Check sheet for the modelled part. Datum: model origin and axes. Units: mm. A direction names the side the tool comes from. Give positions to 0.01 mm unless a question says otherwise; leave off trailing zeros. Write each loop counter-clockwise with the first axis right and the second up, starting at its lowest first coordinate (ties: lowest second). Pieces come first, ordered by that corner, then holes.
from build123d import *

# Parameters (mm, degrees)
BOSS_EXTRUDE1_DEPTH = 12.625


with BuildPart() as part:
    # Sketch1 → Boss-Extrude1 (new, symmetric)
    with BuildSketch(Plane.XY):
        with BuildLine():
            Line((-600, 0), (0, 0))
            ThreePointArc((0, 0), (31, 31), (0, 62))
            Line((0, 62), (-20, 62))
            Line((-20, 62), (-20, 49.4))
            Line((-20, 49.4), (0, 49.4))
            ThreePointArc((0, 49.4), (18.4, 31), (0, 12.6))
            Line((0, 12.6), (-600, 12.6))
            Line((-600, 12.6), (-600, 0))
        make_face()
    extrude(amount=BOSS_EXTRUDE1_DEPTH, both=True)


solid = part.part
1) Sectioned sample at B-B on z = 7.5. Record the boundary of the cut face in (x, y), then the cut area to 3 significant figures.
2) Gauge pin test, flat ends, axial feed: pin 1 (14 mm diameter, centred on y = 58, z = 4.5, fed in from -X); pin 2 (12 mm diameter, centred on y = 35.5, z = 9.5, fed in from +X); pin 3 (1 mm diameter, centred on x = -153, z = -9, fed in from +Y); pin 4 (6 mm diameter, centred on x = -10, z = 1, fed in from -Y). Record the tip position at first contact, or that the pin passes through.
3) Scan lines: L1, parallel to Y at x = -1, z = 1.75; L2, parallel to X at y = 33, z = 7.5; L3, parallel to Y at x = -204.5, z = 4. Record each from-to range of solid material in increasing order.
4) Draft check along Y on faces 3 (the flat face through (-304, 0, 0)), 4 (the flat face through (-10, 49.4, 0)), 5 (the flat face through (-10, 62, 0)). Enter one of: +Y half, -Y half, draft (parallel to the pull), parting line (faces both ways), or undercut.
5) Access from +Z, -Z, +X, -X, +Y, -Y to the whole of each face (thin tool, end or side, straight path). Record for faces 1 (the cylindrical face through (30.993, 30.318, 0.177)), 2 (the flat face through (-20, 56, 0)).
6) Sectioned sample at A-A on x = -6.5. Record the boundary of the cut face in (y, z) (3 decimals).
7) Sectioned sample at C-C on y = 31. Record the boundary of the cut face in (x, z) (3 decimals), then the cut area to 3 significant figures.
8) Sectioned sample at D-D on x = -225. Record the boundary of the cut face in (y, z) (3 decimals).
Answers below:
1. outline: (-600, 0) - (0, 0) arc R31 ccw to (0, 62) - (-20, 62) - (-20, 49.4) - (0, 49.4) arc R18.4 cw to (0, 12.6) - (-600, 12.6) - close
1. area: 8,790 mm2
2. pin 1: stops at x = -20
2. pin 2: stops at x = 31
2. pin 3: stops at y = 12.6
2. pin 4: stops at y = 0
3. L1: y = 0 to 12.6, 49.4 to 62
3. L2: x = 18.29 to 30.94
3. L3: y = 0 to 12.6
4. face 3: -Y half
4. face 4: undercut
4. face 5: +Y half
5. face 1: +Z, -Z, +X
5. face 2: +Z, -Z, -X, +Y
6. outline: (0, -12.625) - (12.6, -12.625) - (12.6, 12.625) - (0, 12.625) - close; (49.4, -12.625) - (62, -12.625) - (62, 12.625) - (49.4, 12.625) - close
7. outline: (18.4, -12.625) - (31, -12.625) - (31, 12.625) - (18.4, 12.625) - close
7. area: 318 mm2
8. outline: (0, -12.625) - (12.6, -12.625) - (12.6, 12.625) - (0, 12.625) - close
